Input: part model. Units: mm. Frame: model coordinates. Give positions to 0.01 mm unless a question says otherwise; leave off trailing zeros. Write each loop counter-clockwise with the first axis right and the second up, starting at its lowest first coordinate (ties: lowest second). Pieces come first, ordered by that corner, then holes.
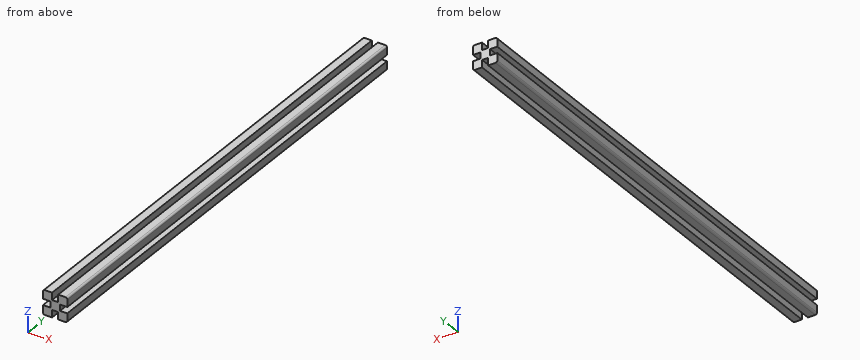
Autodesk Inventor part; units mm, degrees
ref_plane "YZ Plane" through (0, 0, 0) normal (1, 0, 0) x (0, 1, 0)
ref_plane "XZ Plane" through (0, 0, 0) normal (0, 1, 0) x (-1, 0, 0)
ref_plane "XY Plane" through (0, 0, 0) normal (0, 0, 1) x (1, 0, 0)
sketch "Sketch1" plane through (0, 0, 0) normal (0, 1, 0) x (-1, 0, 0)
  line L0 (-5, 20) -> (-5, 8)
  line L1 (5, -20) -> (5, -8)
  line L2 (20, 5) -> (8, 5)
  line L3 (-20, -5) -> (-8, -5)
  line L4 (8, -5) -> (20, -5)
  line L5 (-8, 5) -> (-20, 5)
  line L6 (-5, -8) -> (-5, -20)
  line L7 (5, 8) -> (5, 20)
  arc A0 (-17, 20) -> (-20, 17) centre (-17, 17) ccw
  arc A1 (-20, -17) -> (-17, -20) centre (-17, -17) ccw
  arc A2 (17, -20) -> (20, -17) centre (17, -17) ccw
  arc A3 (20, 17) -> (17, 20) centre (17, 17) ccw
  line L8 (20, 17) -> (20, 5)
  line L9 (20, -5) -> (20, -17)
  line L10 (17, -20) -> (5, -20)
  line L11 (-5, -20) -> (-17, -20)
  line L12 (-20, -17) -> (-20, -5)
  line L13 (-20, 5) -> (-20, 17)
  line L14 (-17, 20) -> (-5, 20)
  line L15 (17, 20) -> (5, 20)
  line L16 (5, 8) -> (-5, 8)
  line L17 (-8, 5) -> (-8, -5)
  line L18 (-5, -8) -> (5, -8)
  line L19 (8, -5) -> (8, 5)
  point P0 (0, 0)
extrude "Extrusion1" add sketch "Sketch1" along normal blind 800
properties part number "column"
Item 1: Ray query, line 1 (Z direction, x = 16.5, y = 326.5); line 2 (Z direction, x = -2, y = 568). Return the intervals inside material, ascending.
Item 2: Pin query (flat end, axial travel): pin 1 (2 mm diameter, centred on y = 604.5, z = -3, fed in from -X); pin 2 (1 mm diameter, centred on x = -3.5, y = 558, fed in from -Z); pin 3 (5 mm diameter, centred on y = 558.5, z = 1.5, fed in from +X). Return the tip coordinate at first contact, or that it passes through.
Item 3: Section A-A (y = 705). Return loops of the section in (x, z), and give its area (3 significant figures).
Solved:
1. line 1: z = -20 to -5, 5 to 20
1. line 2: z = -8 to 8
2. pin 1: stops at x = -8
2. pin 2: stops at z = -8
2. pin 3: stops at x = 8
3. outline: (-20, -17) arc R3 ccw to (-17, -20) - (-5, -20) - (-5, -8) - (5, -8) - (5, -20) - (17, -20) arc R3 ccw to (20, -17) - (20, -5) - (8, -5) - (8, 5) - (20, 5) - (20, 17) arc R3 ccw to (17, 20) - (5, 20) - (5, 8) - (-5, 8) - (-5, 20) - (-17, 20) arc R3 ccw to (-20, 17) - (-20, 5) - (-8, 5) - (-8, -5) - (-20, -5) - close
3. area: 1,110 mm2
